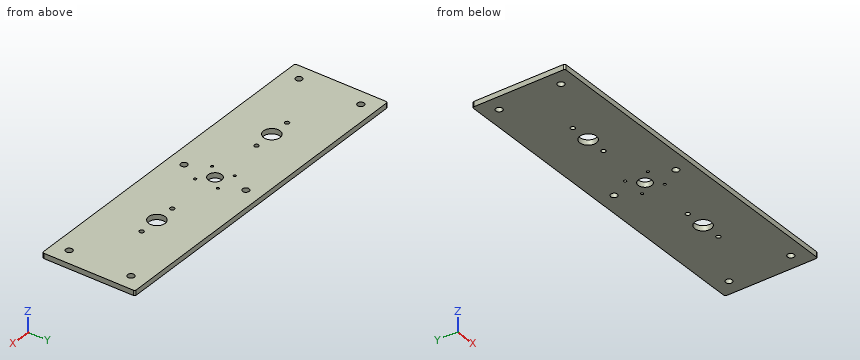
from build123d import *

# Parameters (mm, degrees)
SKETCH1_W                = 330
SKETCH1_H                = 90
BOSS_EXTRUDE1_DEPTH      = 2.5
M6_CLEARANCE_HOLE1_D     = 6.4
M6_CLEARANCE_HOLE1_DEPTH = 10
M6_CLEARANCE_HOLE1_TIP   = 1.922753981
SKETCH3_R                = 8
CUT_EXTRUDE2_DEPTH       = 6
M5X0_8_TAPPED_HOLE1_D    = 4.2
SKETCH4_R                = 6.5
CUT_EXTRUDE3_DEPTH       = 6
M3X0_5_TAPPED_HOLE1_D    = 2.5
FILLET1_R                = 1.5


with BuildPart() as part:
    # Sketch1 → Boss-Extrude1 (new body, symmetric)
    with BuildSketch(Plane.XY):
        Rectangle(SKETCH1_W, SKETCH1_H)
    extrude(amount=BOSS_EXTRUDE1_DEPTH, both=True)

    # M6 Clearance Hole1
    with Locations(Plane.XY.offset(2.5)):
        with Locations((-150, 30), (-150, -30), (0, 30), (0, -30), (150, -30), (150, 30)):
            Hole(M6_CLEARANCE_HOLE1_D / 2, depth=M6_CLEARANCE_HOLE1_DEPTH)
            with Locations((0, 0, -(M6_CLEARANCE_HOLE1_DEPTH + M6_CLEARANCE_HOLE1_TIP / 2))):  # 118° drill point
                Cone(0, M6_CLEARANCE_HOLE1_D / 2, M6_CLEARANCE_HOLE1_TIP, mode=Mode.SUBTRACT)

    # Sketch3 → Cut-Extrude2 (cut, through all)
    with BuildSketch(Plane.XY.offset(2.5)):
        with Locations((-75, -0.6)):
            Circle(SKETCH3_R)
    cut_extrude2 = extrude(amount=-CUT_EXTRUDE2_DEPTH, mode=Mode.SUBTRACT)

    # M5x0.8 Tapped Hole1 (through all)
    with Locations(Plane.XY.offset(2.5)):
        with Locations((-95, -0.6), (-55, -0.6)):
            m5x0_8_tapped_hole1 = Hole(M5X0_8_TAPPED_HOLE1_D / 2)

    # Mirror1: Cut-Extrude2, M5x0.8 Tapped Hole1 across plane
    add(cut_extrude2.mirror(Plane(origin=(0, 0, 0), x_dir=(0, 0, 1), z_dir=(1, 0, 0))), mode=Mode.SUBTRACT)
    add(m5x0_8_tapped_hole1.mirror(Plane(origin=(0, 0, 0), x_dir=(0, 0, 1), z_dir=(1, 0, 0))), mode=Mode.SUBTRACT)

    # Sketch4 → Cut-Extrude3 (cut, through all)
    with BuildSketch(Plane.XY.offset(2.5)):
        Circle(SKETCH4_R)
    extrude(amount=-CUT_EXTRUDE3_DEPTH, mode=Mode.SUBTRACT)

    # M3x0.5 Tapped Hole1 (through all)
    with Locations(Plane.XY.offset(2.5)):
        with Locations((11, 11), (-11, -11), (-11, 11), (11, -11)):
            Hole(M3X0_5_TAPPED_HOLE1_D / 2)

    # Fillet1
    fillet1_edges = [part.edges().sort_by_distance(p)[0] for p in [
        (165, -45, 0),
        (-165, -45, 0),
        (-165, 45, 0),
        (165, 45, 0),
    ]]
    fillet(fillet1_edges, radius=FILLET1_R)


solid = part.part
Model file for the job. Use its own axes, mm. Give positions to 0.01 mm unless a question says otherwise; leave off trailing zeros. Write each loop counter-clockwise with the first axis right and the second up, starting at its lowest first coordinate (ties: lowest second). Pieces come first, ordered by that corner, then holes. Notation, with made-up numbers: (4, 18) -> (24, 18) arc R16 ccw to (24, 46) -> close; hole circle Ø11 at (15.25, 23). An arc over 180 degrees is marked (long way). Write item = value, one per line.
(1) Slice it at A-A, the plane y = -30. Give the cut face in (x, z).
Determined:
outline = (-165, -2.5) -> (-153.2, -2.5) -> (-153.2, 2.5) -> (-165, 2.5) -> close; (-146.8, -2.5) -> (-3.2, -2.5) -> (-3.2, 2.5) -> (-146.8, 2.5) -> close; (3.2, -2.5) -> (146.8, -2.5) -> (146.8, 2.5) -> (3.2, 2.5) -> close; (153.2, -2.5) -> (165, -2.5) -> (165, 2.5) -> (153.2, 2.5) -> close
(2) Slice it at C-C, the plane z = -1.3. Give the number of separate pieces and of enclosed holes in the cut face, then the cut area to 3 significant figures.
Determined:
separate_pieces = 1
enclosed_holes = 17
area = 28,900 mm2
(3) Flat gauge pins, fed straight in: P1, Ø5.5, axis at x = -95, y = -0.6, coming from the +Z side; P2, Ø5, axis at x = -150, y = 30, coming from the +Z side. Where does each tip first touch, or does it go through?
Determined:
P1 = 2.5
P2 = through
(4) Slice it at B-B, the plane x = 0. Give the cut face in (y, z), then the cut area to 3 significant figures.
Determined:
outline = (-45, -2.5) -> (-33.2, -2.5) -> (-33.2, 2.5) -> (-45, 2.5) -> close; (-26.8, -2.5) -> (-6.5, -2.5) -> (-6.5, 2.5) -> (-26.8, 2.5) -> close; (6.5, -2.5) -> (26.8, -2.5) -> (26.8, 2.5) -> (6.5, 2.5) -> close; (33.2, -2.5) -> (45, -2.5) -> (45, 2.5) -> (33.2, 2.5) -> close
area = 321 mm2
(5) Slice it at D-D, the plane x = 75. Give the cut face in (y, z), then the cut area to 3 significant figures.
Determined:
outline = (-45, -2.5) -> (-8.6, -2.5) -> (-8.6, 2.5) -> (-45, 2.5) -> close; (7.4, -2.5) -> (45, -2.5) -> (45, 2.5) -> (7.4, 2.5) -> close
area = 370 mm2
(6) Probe line 1 along Y through (x, z) = (150, -0.65); line 2 along Y through (x, z) = (1, 1.2); line 3 along Y through (x, z) = (-55, 0.05). List the from-to ranges inside material, lowest first.
Determined:
line_1 = -45 to -33.2, -26.8 to 26.8, 33.2 to 45
line_2 = -45 to -33.04, -26.96 to -6.42, 6.42 to 26.96, 33.04 to 45
line_3 = -45 to -2.7, 1.5 to 45
